from build123d import *

# Parameters (mm, degrees)
BOSS_EXTRUDE1_DEPTH = 13
SKETCH2_R           = 1.6
SKETCH2_R_2         = 1.611537585
CUT_EXTRUDE1_DEPTH  = 20
SKETCH3_R           = 3
CUT_EXTRUDE2_DEPTH  = 1
SKETCH4_R           = 2.9
CUT_EXTRUDE3_DEPTH  = 1
SKETCH5_W           = 1
SKETCH5_H           = 7.5
BOSS_EXTRUDE2_DEPTH = 1
LPATTERN1_COUNT     = 7
LPATTERN1_PITCH     = 2
SKETCH6_W           = 1
SKETCH6_H           = 7.5
BOSS_EXTRUDE3_DEPTH = 1
LPATTERN2_COUNT     = 7
LPATTERN2_PITCH     = 2
CHAMFER1_SIZE       = 10
FILLET1_R           = 4


with BuildPart() as part:
    # Sketch1 → Boss-Extrude1 (new body)
    with BuildSketch(Plane.XY.offset(98.171636097)):
        Polygon((31.214370899, 78.263460463), (35.214370899, 78.263460463), (35.214370899, 66.863460463), (35.214370899, 63.263460463), (26.214370899, 63.263460463), (26.214370899, 49.763460463), (23.214370899, 49.763460463), (23.214370899, 63.263460463), (23.214370899, 63.763460463), (31.214370899, 63.763460463), align=None)
    extrude(amount=-BOSS_EXTRUDE1_DEPTH)

    # Sketch2 → Cut-Extrude1 (cut)
    with BuildSketch(Plane(origin=(35.214370899, 0, 0), x_dir=(0, 0, -1), z_dir=(1, 0, 0))):
        with Locations((-91.671636097, 75.863460463)):
            Circle(SKETCH2_R)
        with Locations((-91.671636097, 54.263460463)):
            Circle(SKETCH2_R_2)
    extrude(amount=-CUT_EXTRUDE1_DEPTH, mode=Mode.SUBTRACT)

    # Sketch3 → Cut-Extrude2 (cut)
    with BuildSketch(Plane.ZY.offset(-23.214370899)):
        with Locations((91.671636097, 54.263460463)):
            Circle(SKETCH3_R)
    extrude(amount=-CUT_EXTRUDE2_DEPTH, mode=Mode.SUBTRACT)

    # Sketch4 → Cut-Extrude3 (cut)
    with BuildSketch(Plane.ZY.offset(-31.214370899)):
        with Locations((91.671636097, 75.863460463)):
            Circle(SKETCH4_R)
    extrude(amount=-CUT_EXTRUDE3_DEPTH, mode=Mode.SUBTRACT)

    # Sketch5 → Boss-Extrude2 (add)
    with BuildSketch(Plane(origin=(35.214370899, 0, 0), x_dir=(0, 0, -1), z_dir=(1, 0, 0))):
        with Locations((-97.671636097, 70.113460463)):
            Rectangle(SKETCH5_W, SKETCH5_H)
    boss_extrude2 = extrude(amount=BOSS_EXTRUDE2_DEPTH)

    # LPattern1: Boss-Extrude2 ×7
    with Locations(*[(0, 0, -i * LPATTERN1_PITCH) for i in range(1, LPATTERN1_COUNT)]):
        add(boss_extrude2)

    # Sketch6 → Boss-Extrude3 (add)
    with BuildSketch(Plane(origin=(26.214370899, 0, 0), x_dir=(0, 0, -1), z_dir=(1, 0, 0))):
        with Locations((-97.671636097, 60.113460463)):
            Rectangle(SKETCH6_W, SKETCH6_H)
    boss_extrude3 = extrude(amount=BOSS_EXTRUDE3_DEPTH)

    # LPattern2: Boss-Extrude3 ×7
    with Locations(*[(0, 0, -i * LPATTERN2_PITCH) for i in range(1, LPATTERN2_COUNT)]):
        add(boss_extrude3)

    # Chamfer1
    # the kernel refuses this chamfer: 10 mm, written as the material it adds along each edge
    with BuildSketch(Plane(origin=(31.214370899, 63.763460463, 98.171636097), x_dir=(0.027495876610585647, 0.9996219169112968, 0), z_dir=(0, 0, -1))) as chamfer1_piece_1_section:
        Polygon((CHAMFER1_SIZE * 0.999621916911, -CHAMFER1_SIZE * 0.0274958766106), (-CHAMFER1_SIZE * 0.0274958766106, -CHAMFER1_SIZE * 0.999621916911), (0, 0), align=None)
    chamfer1_piece_1 = extrude(amount=13, mode=Mode.PRIVATE)
    chamfer1_piece_1 = chamfer1_piece_1 - Plane(origin=(28.210743814, 75.863460463, 91.671636097), x_dir=(0, 0, 1), z_dir=(-1, 0, 0)) * Cylinder(2.9, 66, mode=Mode.PRIVATE)
    chamfer1_piece_1 = split(chamfer1_piece_1, bisect_by=Plane(origin=(23.214370899, 67.201513325, 91.671636099), z_dir=(1, 0, 0)), keep=Keep.TOP, mode=Mode.PRIVATE)
    add(chamfer1_piece_1)

    # Fillet1
    fillet1_edges = [part.edges().sort_by_distance(p)[0] for p in [
        (24.714370899, 49.763460463, 98.171636097),
    ]]
    fillet(fillet1_edges, radius=FILLET1_R)


solid = part.part
Geometry: final body of the model. Coordinates: model frame, mm. A direction names the side the tool comes from. Coordinates: 2 decimals unless noted, no trailing zeros. Order: outer loops, then holes, each group sorted by start corner. A loop starts at its lowest first (then second) coordinate and runs counter-clockwise, first axis right, second up.
1) Section A-A (z = 92.5). Return loops of the section in (x, y).
Result sheet:
outline: (23.21, 49.76) - (26.21, 49.76) - (26.21, 52.88) - (24.21, 52.88) - (24.21, 51.38) - (23.21, 51.38) - close; (23.21, 57.15) - (24.21, 57.15) - (24.21, 55.65) - (26.21, 55.65) - (26.21, 63.26) - (35.21, 63.26) - (35.21, 74.49) - (32.21, 74.49) - (32.21, 73.08) - (30.54, 73.08) - (23.21, 65.76) - close; (32.21, 77.23) - (35.21, 77.23) - (35.21, 78.26) - (32.21, 78.26) - close
2) Section D-D (y = 67.75). Return loops of the section in (x, z), then the cut area to 3 significant figures.
Result sheet:
outline: (25.2, 85.17) - (36.21, 85.17) - (36.21, 86.17) - (35.21, 86.17) - (35.21, 87.17) - (36.21, 87.17) - (36.21, 88.17) - (35.21, 88.17) - (35.21, 89.17) - (36.21, 89.17) - (36.21, 90.17) - (35.21, 90.17) - (35.21, 91.17) - (36.21, 91.17) - (36.21, 92.17) - (35.21, 92.17) - (35.21, 93.17) - (36.21, 93.17) - (36.21, 94.17) - (35.21, 94.17) - (35.21, 95.17) - (36.21, 95.17) - (36.21, 96.17) - (35.21, 96.17) - (35.21, 97.17) - (36.21, 97.17) - (36.21, 98.17) - (25.2, 98.17) - close
area: 137 mm2
3) Section C-C (x = 24.75). Return loops of the section in (y, z), then the cut area to 3 significant figures.
Result sheet:
outline: (49.76, 85.17) - (67.3, 85.17) - (67.3, 98.17) - (53.76, 98.17) arc R4 ccw to (49.76, 94.17) - close; hole circle Ø3.22 at (54.26, 91.67)
area: 216 mm2
4) Set-up query: faces 5 (the flat face through (27, 60, 86.172)), 6 (the flat face through (27, 56.363, 88)), 7 (the flat face through (36, 70, 94.172)). Return all of +Z, -Z, +X, -X, +Y, -Y with unobstructed straight access to the full face (end or side cutting, diameter ignored); none if empty.
Result sheet:
face 5: +X, -Y
face 6: +Z, -Z, +X, -Y
face 7: +X, +Y, -Y
5) Ray query, probe 1 along Y at (x, z) = (32.5, 89); probe 2 along X at (y, z) = (56.25, 93.5); probe 3 along Y at (x, z) = (34, 90.25). Return the intervals inside material, ascending.
Result sheet:
probe 1: y = 63.26 to 78.26
probe 2: x = 24.21 to 26.21
probe 3: y = 63.26 to 75.13, 76.6 to 78.26
6) Draft query along Z for faces 1 (the flat face through (30, 66, 98.172)), 2 (the cylindrical face through (31.667, 72.965, 91.568)), 3 (the flat face through (27, 60, 90.172)), 4 (the flat face through (36.214, 70, 94)). Return one class per face: released by +Z, released by -Z, zero draft, split by the parting line, or undercut.
Result sheet:
face 1: released by +Z
face 2: undercut
face 3: undercut
face 4: zero draft
7) First-contact query: P1, Ø0.5, axis at y = 58.5, z = 93.5, coming from the +X side; P2, Ø0.5, axis at x = 36, z = 85.5, coming from the +Y side; P3, Ø0.5, axis at x = 26.5, z = 95.5, coming from the -Y side. Flat tips, straight axial feed; report the tip coordinate or a pass-through.
Result sheet:
P1: stops at x = 27.21
P2: stops at y = 73.86
P3: stops at y = 56.36
8) Section B-B (y = 75.5). Return loops of the section in (x, z).
Result sheet:
outline: (31.21, 85.17) - (35.21, 85.17) - (35.21, 90.11) - (32.21, 90.11) - (32.21, 88.79) - (31.21, 88.79) - close; (31.21, 94.55) - (32.21, 94.55) - (32.21, 93.23) - (35.21, 93.23) - (35.21, 98.17) - (31.21, 98.17) - close
